Verification items for this drawing (mm, ordinates from the low corner). A direction names the side the tool comes from. Coordinates: 2 decimals unless noted, no trailing zeros. Loops run counter-clockwise (first coordinate to the right, second up) from the corner with the lowest first, then second, coordinate; pieces in that order, holes last. Notation, with made-up numbers: M 27,88.5 L 61,88.5 A24 ccw 61,120.5 Z; hole C 81,-5.75 d5. An arc over 180 degrees is marked long. One line per question, with ' | ' between items. Start each with the question number.
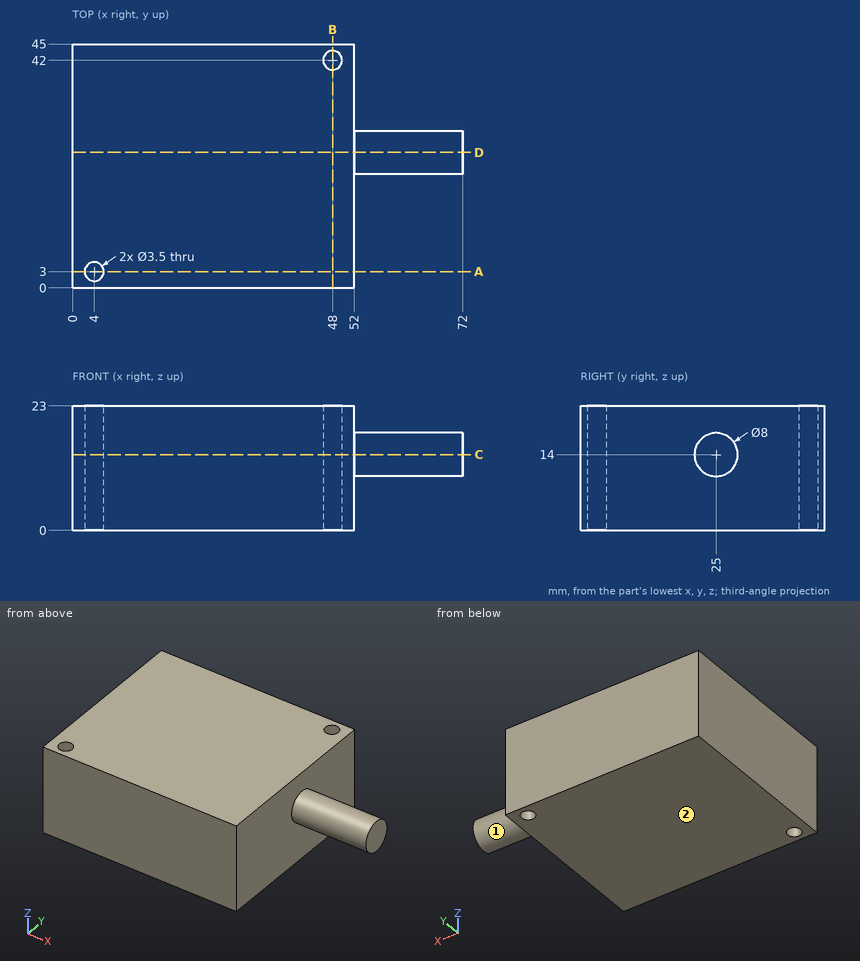
1. Tool access check on the marked faces 1 and 2. Record the directions out of +Z, -Z, +X, -X, +Y, -Y that give a thin tool (end or side, any length) a straight path to the whole face; none if there is none.
2. Sectioned sample at C-C (z = 14). Record the cut outline in (x, y).
3. Thickness scan on line 1 (Y direction, x = 4, z = 7); line 2 (X direction, y = 38, z = 5); line 3 (X direction, y = 43, z = 1.25). Record the ranges inside material, lowest first.
4. Sectioned sample at B-B (x = 48). Record the cut outline in (y, z), and give its area (4 significant figures).
5. Depth check by flat-ended pin: pin 1 Ø6 at (y, z) = (21, 3) entering from +X. Enter the tip coordinate at first touch or a pass-through.
6. Sectioned sample at A-A (y = 3). Record the cut outline in (x, z).
7. Sectioned sample at D-D (y = 25). Record the cut outline in (x, z).
Result:
1) face 1: +X | face 2: -Z, +X, -X, +Y, -Y
2) outline: M 0,0 L 52,0 L 52,21 L 72,21 L 72,29 L 52,29 L 52,45 L 0,45 Z; hole C 4,3 d3.5; hole C 48,42 d3.5
3) line 1: y = 0 to 1.25, 4.75 to 45 | line 2: x = 0 to 52 | line 3: x = 0 to 46.56, 49.44 to 52
4) outline: M 0,0 L 40.25,0 L 40.25,23 L 0,23 Z; M 43.75,0 L 45,0 L 45,23 L 43.75,23 Z | area: 954.5 mm2
5) pin 1: stops at x = 52
6) outline: M 0,0 L 2.25,0 L 2.25,23 L 0,23 Z; M 5.75,0 L 52,0 L 52,23 L 5.75,23 Z
7) outline: M 0,0 L 52,0 L 52,10 L 72,10 L 72,18 L 52,18 L 52,23 L 0,23 Z
